CAD build for the part. Positions are in the model's coordinates, mm. A direction names the side the tool comes from. Give positions to 0.01 mm unless a question says otherwise; leave off trailing zeros. Order: outer loops, then holes, each group sorted by start corner. A loop starts at its lowest first (then second) coordinate and runs counter-clockwise, first axis right, second up. Notation, with made-up numbers: (8, -40) -> (64, -40) arc R18 ccw to (64, -6) -> close; hole circle Ø11 at (9.5, 3). An arc over 180 degrees is marked (long way). Answer as CSV lines item,"result".
Autodesk Inventor part; units mm, degrees
ref_plane "YZ Plane" through (0, 0, 0) normal (1, 0, 0) x (0, 1, 0)
ref_plane "XZ Plane" through (0, 0, 0) normal (0, 1, 0) x (-1, 0, 0)
ref_plane "XY Plane" through (0, 0, 0) normal (0, 0, 1) x (1, 0, 0)
sketch "Sketch1" plane through (0, 0, 0) normal (0, 1, 0) x (-1, 0, 0)
  line L0 (-63.5, -111) -> (63.5, -111)
  line L1 (63.5, -111) -> (63.5, 111)
  line L2 (63.5, 111) -> (-63.5, 111)
  line L3 (-63.5, 111) -> (-63.5, -111)
  line L4 (-63.5, -111) -> (63.5, 111) construction
  line L5 (63.5, -111) -> (-63.5, 111) construction
  point P0 (0, 0)
  dimension "d0" = 127
  dimension "d1" = 222
extrude "Extrusion1" add sketch "Sketch1" along normal blind 19.05
sketch "Sketch12" plane through (0, 19.05, 0) normal (0, 1, 0) x (1, 0, 0)
  line L0 (63.5, -111) -> (63.5, 111)
  line L1 (-16.5, -104.15) -> (63.5, -104.15)
  line L2 (63.5, -104.15) -> (63.5, -105.65)
  line L3 (63.5, -105.65) -> (-16.5, -105.65)
  circle A0 centre (33, -60.25) radius 1.2295
  circle A1 centre (33, -47.45) radius 1.2295
  arc A2 (-16.5, -104.15) -> (-16.5, -105.65) centre (-16.5, -104.9) ccw
  circle A3 centre (-33, -9.45) radius 1.2295
  circle A4 centre (-33, -60.25) radius 1.2295
  circle A5 centre (33, -98.25) radius 1.2295
  line L4 (-16.5, -53.35) -> (63.5, -53.35)
  line L5 (63.5, -53.35) -> (63.5, -54.85)
  line L6 (63.5, -54.85) -> (-16.5, -54.85)
  arc A6 (-16.5, -53.35) -> (-16.5, -54.85) centre (-16.5, -54.1) ccw
  line L7 (-16.5, -2.55) -> (63.5, -2.55)
  line L8 (63.5, -2.55) -> (63.5, -4.05)
  line L9 (63.5, -4.05) -> (-16.5, -4.05)
  arc A7 (-16.5, -2.55) -> (-16.5, -4.05) centre (-16.5, -3.3) ccw
  line L10 (-16.5, 48.25) -> (63.5, 48.25)
  line L11 (63.5, 48.25) -> (63.5, 46.75)
  line L12 (63.5, 46.75) -> (-16.5, 46.75)
  arc A8 (-16.5, 48.25) -> (-16.5, 46.75) centre (-16.5, 47.5) ccw
  point P0 (0, 0)
  point P1 (63.5, -60.2)
  point P2 (63.5, -9.4)
  point P3 (63.5, 41.4)
  dimension "d156" = 1.5
  dimension "d157" = 12.8
  dimension "d159" = 0.75
  dimension "d160" = 80
  dimension "d161" = 50.8
  dimension "d162" = 5.9
  dimension "d165" = 50.8
extrude "Extrusion7" cut sketch "Sketch12" against normal blind 16.5 contours L3 A2 L1 L0 | L6 A6 L4 L0 | L9 A7 L7 L0 | L12 A8 L10 L0
sketch "Sketch13" plane through (63.5, 0, 111) normal (1, 0, 0) x (0, 0, -1)
  line L0 (0, 0) -> (222, 0)
  line L1 (0, 0) -> (0, 19.05)
  line L2 (56.15, 2.55) -> (56.15, 19.05)
  line L3 (5.35, 2.55) -> (5.35, 19.05)
  point P0 (111, 0)
  point P1 (25.91, 12.3)
  point P2 (40.91, 12.3)
  point P3 (0, 17.05)
  point P4 (56.65, 17.05)
  point P5 (5.85, 17.05)
  point P6 (76.71, 12.3)
  point P7 (91.71, 12.3)
  point P8 (127.51, 12.3)
  point P9 (142.51, 12.3)
  point P10 (178.31, 12.3)
  point P11 (193.31, 12.3)
  point P12 (56.15, 19.05)
  point P13 (5.35, 19.05)
  dimension "d176" = 50.8
  dimension "d173" = 12.3
  dimension "d174" = 15
  dimension "d175" = 25.91
  dimension "d179" = 50.8
hole "Hole7" at (63.5, 12.3, 85.09) at (63.5, 12.3, 70.09) at (63.5, 12.3, 34.29) at (63.5, 12.3, 19.29) at (63.5, 12.3, -16.51) at (63.5, 12.3, -31.51) at (63.5, 12.3, -67.31) at (63.5, 12.3, -82.31) direction (-1, 0, 0) diameter 2.459 depth 8.8 tip angle 118
sketch "Sketch14" plane through (63.5, 0, 111) normal (1, 0, 0) x (0, 0, -1)
  line L0 (6.85, 19.05) -> (6.85, 2.55)
  arc A0 (14.85, 19.05) -> (6.85, 11.05) centre (14.85, 11.05) ccw
  line L1 (14.85, 11.05) -> (14.85, 19.05) construction
  line L2 (14.85, 11.05) -> (6.85, 11.05) construction
  line L3 (6.85, 19.05) -> (56.15, 19.05)
  line L4 (14.85, 19.05) -> (6.85, 19.05)
  line L5 (6.85, 19.05) -> (6.85, 11.05)
  arc A1 (65.65, 19.05) -> (57.65, 11.05) centre (65.65, 11.05) ccw
  line L6 (65.65, 19.05) -> (57.65, 19.05)
  line L7 (57.65, 19.05) -> (57.65, 11.05)
  arc A2 (116.45, 19.05) -> (108.45, 11.05) centre (116.45, 11.05) ccw
  line L8 (116.45, 19.05) -> (108.45, 19.05)
  line L9 (108.45, 19.05) -> (108.45, 11.05)
  arc A3 (167.25, 19.05) -> (159.25, 11.05) centre (167.25, 11.05) ccw
  line L10 (167.25, 19.05) -> (159.25, 19.05)
  line L11 (159.25, 19.05) -> (159.25, 11.05)
  point P0 (111, 0)
  dimension "d191" = 90
  dimension "d192" = 8
  dimension "d193" = 8
  dimension "d198" = 50.8
extrude "Extrusion8" cut sketch "Sketch14" against normal blind 79
extrude "Extrusion10" add sketch "Sketch14" against normal blind 50
sketch "Sketch15" plane through (0, 19.05, 0) normal (0, 1, 0) x (1, 0, 0)
  arc A0 (55.5, -104.15) -> (63.5, -96.15) centre (55.5, -96.15) ccw
  line L0 (55.5, -96.15) -> (55.5, -104.15) construction
  line L1 (55.5, -96.15) -> (63.5, -96.15) construction
  line L2 (-15.5, -104.15) -> (63.5, -104.15)
  line L3 (63.5, -96.15) -> (63.5, -54.85)
  line L4 (-16.5, -104.15) -> (63.5, -104.15)
  line L5 (55.5, -104.15) -> (63.5, -104.15)
  line L6 (63.5, -104.15) -> (63.5, -96.15)
  arc A1 (55.5, -53.35) -> (63.5, -45.35) centre (55.5, -45.35) ccw
  line L7 (63.5, -53.35) -> (63.5, -45.35)
  line L8 (55.5, -53.35) -> (63.5, -53.35)
  arc A2 (55.5, -2.55) -> (63.5, 5.45) centre (55.5, 5.45) ccw
  line L9 (63.5, -2.55) -> (63.5, 5.45)
  line L10 (55.5, -2.55) -> (63.5, -2.55)
  arc A3 (55.5, 48.25) -> (63.5, 56.25) centre (55.5, 56.25) ccw
  line L11 (63.5, 48.25) -> (63.5, 56.25)
  line L12 (55.5, 48.25) -> (63.5, 48.25)
  point P0 (0, 0)
  point P1 (63.5, 56.25)
  point P2 (63.5, 5.45)
  dimension "d203" = 90
  dimension "d204" = 8
  dimension "d207" = 50.8
extrude "Extrusion9" cut sketch "Sketch15" against normal up to surface (16.5 mm away)
sketch "Sketch16" plane through (0, 19.05, 0) normal (0, 1, 0) x (1, 0, 0)
  line L0 (-15.5, -96.15) -> (13.5, -96.15)
  line L1 (13.5, -104.15) -> (13.5, -96.15)
  point P0 (0, 0)
  point P1 (7.5, -75.85)
  point P2 (-7.5, -75.85)
  point P3 (-16.5, -96.15)
  point P4 (-7.5, -25.05)
  point P5 (7.5, -25.05)
  point P6 (-7.5, 25.75)
  point P7 (7.5, 25.75)
  point P8 (-7.5, 76.55)
  point P9 (7.5, 76.55)
  dimension "d216" = 20.3
  dimension "d217" = 15
  dimension "d218" = 6
  dimension "d221" = 50.8
hole "Hole8" at (-7.5, 19.05, 25.05) at (-7.5, 19.05, -25.75) at (7.5, 19.05, -25.75) at (-7.5, 19.05, -76.55) at (7.5, 19.05, -76.55) at (7.5, 19.05, 75.85) at (-7.5, 19.05, 75.85) at (7.5, 19.05, 25.05) direction (0, -1, 0) diameter 2 end through all
sketch "Sketch17" plane through (0, 19.05, 0) normal (0, 1, 0) x (1, 0, 0)
  line L0 (63.5, -111) -> (63.5, 111)
  line L1 (63.5, -111) -> (-19.9113, -111)
  line L2 (-19.9113, -111) -> (-19.9113, -56.7947)
  line L3 (-19.9113, -56.7947) -> (63.5, -56.7947)
  line L4 (63.5, -56.7947) -> (63.5, -111)
  line L5 (-63.5, 111) -> (-63.5, -111)
  line L6 (-19.9113, -111) -> (-63.5, -111)
  line L7 (-63.5, -111) -> (-63.5, 111)
  line L8 (-63.5, 111) -> (63.5, 111)
  point P0 (0, 0)
extrude "Extrusion11" cut sketch "Sketch17" against normal through all contours L3 L2 L6 L5 L8 L0
properties part number "Tamale Assembly Plate FLEX V1 Print Section"
1) Which spindle directions (+Z, -Z, +X, -X, +Y, -Y) get a long thin tool onto all of the face, cutting with end or side? Do faces 1 (the flat face through (13.5, 17, 103)), 2 (the flat face through (27, 9, 104.15)), 3 (the conical face through (54.09, 12.48, 84.98)). Say none if no direction does.
Data:
face 1,"+Y"
face 2,"+X, +Y"
face 3,"+X"
2) Pull direction Z, two halves, no side cores. Call faces 4 (the flat face through (21, 9, 111)), 5 (the cylindrical face through (59.04, 12.25, 86.32)), 6 (the flat face through (63.5, 9, 78)): pulls with the +Z half, pulls with the -Z half, needs draft (parallel to the pull), parting line crosses it, or undercut.
Data:
face 4,"pulls with the +Z half"
face 5,"undercut"
face 6,"needs draft"
3) Wall check: line 1 along Z through (x, y) = (-7.5, 11); line 2 along Z through (x, y) = (28, 10); line 3 along X through (y, z) = (12.75, 75.85). Give the ranges that are in metal, low to high. Write a range as [from, to].
Data:
line 1,"z = [56.79, 74.85], [76.85, 104.15], [105.65, 111]"
line 2,"z = [56.79, 104.15], [105.65, 111]"
line 3,"x = [-19.91, -8.5], [-6.5, 6.5], [8.5, 63.5]"
4) Band-saw the part on B-B, the plane z = 75.85. Write the cut outline in (x, y).
Data:
outline,"(-19.91, 0) -> (-8.5, 0) -> (-8.5, 19.05) -> (-19.91, 19.05) -> close; (-6.5, 0) -> (6.5, 0) -> (6.5, 19.05) -> (-6.5, 19.05) -> close; (8.5, 0) -> (63.5, 0) -> (63.5, 19.05) -> (8.5, 19.05) -> close"
5) Pin check, flat tips, straight feed: P1, Ø1.5, axis at y = 12.3, z = 70.09, coming from the +X side; P2, Ø2.5, axis at y = 13.5, z = 102, coming from the +X side. Stop position of each tip, or through.
Data:
P1,"stops at x = 54.41"
P2,"stops at x = 62.05"
6) Band-saw the part on C-C, the plane y = 10. Write the cut outline in (x, z).
Data:
outline,"(-19.91, 56.79) -> (63.5, 56.79) -> (63.5, 96.15) arc R8 ccw to (55.5, 104.15) -> (-16.5, 104.15) arc R0.75 cw to (-16.5, 105.65) -> (63.5, 105.65) -> (63.5, 111) -> (-19.91, 111) -> close; hole circle Ø2 at (-7.5, 75.85); hole circle Ø2 at (7.5, 75.85)"
7) Band-saw the part on D-D, the plane x = 3. Write the cut outline in (y, z).
Data:
outline,"(0, 56.79) -> (19.05, 56.79) -> (19.05, 96.15) arc R8 ccw to (11.05, 104.15) -> (2.55, 104.15) -> (2.55, 105.65) -> (19.05, 105.65) -> (19.05, 111) -> (0, 111) -> close"
8) Band-saw the part on A-A, the plane x = -7.5. Write the cut outline in (y, z).
Data:
outline,"(0, 56.79) -> (19.05, 56.79) -> (19.05, 74.85) -> (0, 74.85) -> close; (0, 76.85) -> (19.05, 76.85) -> (19.05, 96.15) arc R8 ccw to (11.05, 104.15) -> (2.55, 104.15) -> (2.55, 105.65) -> (19.05, 105.65) -> (19.05, 111) -> (0, 111) -> close"
